from build123d import *

# Parameters (mm, degrees)
SKETCH1_R                 = 2.1
BOSS_EXTRUDE1_DEPTH       = 400
M5X0_8_TAPPED_HOLE1_D     = 4.2
M5X0_8_TAPPED_HOLE1_DEPTH = 14
M5X0_8_TAPPED_HOLE1_TIP   = 1.2618073
M5X0_8_TAPPED_HOLE2_D     = 4.2
M5X0_8_TAPPED_HOLE2_DEPTH = 14
M5X0_8_TAPPED_HOLE2_TIP   = 1.2618073


with BuildPart() as part:
    # Sketch1 → Boss-Extrude1 (new body)
    with BuildSketch(Plane(origin=(0, 0, -400), x_dir=(-1, 0, 0), z_dir=(0, 0, -1))):
        with BuildLine():
            Line((10, -17), (10, -3))
            Line((10, -3), (8, -3))
            Line((8, -3), (8, -6))
            Line((8, -6), (7.060660172, -6))
            Line((7.060660172, -6), (4, -2.939339828))
            Line((4, -2.939339828), (4, -0.519615242))
            Line((4, -0.519615242), (3.7, 0))
            Line((3.7, 0), (4, 0.519615242))
            Line((4, 0.519615242), (4, 2.939339828))
            Line((4, 2.939339828), (7.060660172, 6))
            Line((7.060660172, 6), (8, 6))
            Line((8, 6), (8, 3))
            Line((8, 3), (10, 3))
            Line((10, 3), (10, 17))
            Line((10, 17), (8, 17))
            Line((8, 17), (8, 14))
            Line((8, 14), (7.060660172, 14))
            Line((7.060660172, 14), (4, 17.060660172))
            Line((4, 17.060660172), (4, 19.480384758))
            Line((4, 19.480384758), (3.7, 20))
            Line((3.7, 20), (4, 20.519615242))
            Line((4, 20.519615242), (4, 22.939339828))
            Line((4, 22.939339828), (7.060660172, 26))
            Line((7.060660172, 26), (8, 26))
            Line((8, 26), (8, 23))
            Line((8, 23), (10, 23))
            Line((10, 23), (10, 29))
            ThreePointArc((10, 29), (9.707106781, 29.707106781), (9, 30))
            Line((9, 30), (3, 30))
            Line((3, 30), (3, 28))
            Line((3, 28), (6, 28))
            Line((6, 28), (6, 27.060660172))
            Line((6, 27.060660172), (2.939339828, 24))
            Line((2.939339828, 24), (0.519615242, 24))
            Line((0.519615242, 24), (0, 23.7))
            Line((0, 23.7), (-0.519615242, 24))
            Line((-0.519615242, 24), (-2.939339828, 24))
            Line((-2.939339828, 24), (-6, 27.060660172))
            Line((-6, 27.060660172), (-6, 28))
            Line((-6, 28), (-3, 28))
            Line((-3, 28), (-3, 30))
            Line((-3, 30), (-9, 30))
            ThreePointArc((-9, 30), (-9.707106781, 29.707106781), (-10, 29))
            Line((-10, 29), (-10, 23))
            Line((-10, 23), (-8, 23))
            Line((-8, 23), (-8, 26))
            Line((-8, 26), (-7.060660172, 26))
            Line((-7.060660172, 26), (-4, 22.939339828))
            Line((-4, 22.939339828), (-4, 20.519615242))
            Line((-4, 20.519615242), (-3.7, 20))
            Line((-3.7, 20), (-4, 19.480384758))
            Line((-4, 19.480384758), (-4, 17.060660172))
            Line((-4, 17.060660172), (-7.060660172, 14))
            Line((-7.060660172, 14), (-8, 14))
            Line((-8, 14), (-8, 17))
            Line((-8, 17), (-10, 17))
            Line((-10, 17), (-10, 3))
            Line((-10, 3), (-8, 3))
            Line((-8, 3), (-8, 6))
            Line((-8, 6), (-7.060660172, 6))
            Line((-7.060660172, 6), (-4, 2.939339828))
            Line((-4, 2.939339828), (-4, 0.519615242))
            Line((-4, 0.519615242), (-3.7, 0))
            Line((-3.7, 0), (-4, -0.519615242))
            Line((-4, -0.519615242), (-4, -2.939339828))
            Line((-4, -2.939339828), (-7.060660172, -6))
            Line((-7.060660172, -6), (-8, -6))
            Line((-8, -6), (-8, -3))
            Line((-8, -3), (-10, -3))
            Line((-10, -3), (-10, -17))
            Line((-10, -17), (-8, -17))
            Line((-8, -17), (-8, -14))
            Line((-8, -14), (-7.060660172, -14))
            Line((-7.060660172, -14), (-4, -17.060660172))
            Line((-4, -17.060660172), (-4, -19.480384758))
            Line((-4, -19.480384758), (-3.7, -20))
            Line((-3.7, -20), (-4, -20.519615242))
            Line((-4, -20.519615242), (-4, -22.939339828))
            Line((-4, -22.939339828), (-7.060660172, -26))
            Line((-7.060660172, -26), (-8, -26))
            Line((-8, -26), (-8, -23))
            Line((-8, -23), (-10, -23))
            Line((-10, -23), (-10, -29))
            ThreePointArc((-10, -29), (-9.707106781, -29.707106781), (-9, -30))
            Line((-9, -30), (-3, -30))
            Line((-3, -30), (-3, -28))
            Line((-3, -28), (-6, -28))
            Line((-6, -28), (-6, -27.060660172))
            Line((-6, -27.060660172), (-2.939339828, -24))
            Line((-2.939339828, -24), (-0.519615242, -24))
            Line((-0.519615242, -24), (0, -23.7))
            Line((0, -23.7), (0.519615242, -24))
            Line((0.519615242, -24), (2.939339828, -24))
            Line((2.939339828, -24), (6, -27.060660172))
            Line((6, -27.060660172), (6, -28))
            Line((6, -28), (3, -28))
            Line((3, -28), (3, -30))
            Line((3, -30), (9, -30))
            ThreePointArc((9, -30), (9.707106781, -29.707106781), (10, -29))
            Line((10, -29), (10, -23))
            Line((10, -23), (8, -23))
            Line((8, -23), (8, -26))
            Line((8, -26), (7.060660172, -26))
            Line((7.060660172, -26), (4, -22.939339828))
            Line((4, -22.939339828), (4, -20.519615242))
            Line((4, -20.519615242), (3.7, -20))
            Line((3.7, -20), (4, -19.480384758))
            Line((4, -19.480384758), (4, -17.060660172))
            Line((4, -17.060660172), (7.060660172, -14))
            Line((7.060660172, -14), (8, -14))
            Line((8, -14), (8, -17))
            Line((8, -17), (10, -17))
        make_face()
        Circle(SKETCH1_R, mode=Mode.SUBTRACT)
        with Locations((0, -20)):
            Circle(SKETCH1_R, mode=Mode.SUBTRACT)
        with Locations((0, 20)):
            Circle(SKETCH1_R, mode=Mode.SUBTRACT)
        Polygon((6.939339828, -8), (8, -8), (8, -12), (6.939339828, -12), (2.939339828, -16), (-2.939339828, -16), (-6.939339828, -12), (-8, -12), (-8, -8), (-6.939339828, -8), (-2.939339828, -4), (2.939339828, -4), align=None, mode=Mode.SUBTRACT)
        Polygon((8, 12), (8, 8), (6.939339828, 8), (2.939339828, 4), (-2.939339828, 4), (-6.939339828, 8), (-8, 8), (-8, 12), (-6.939339828, 12), (-2.939339828, 16), (2.939339828, 16), (6.939339828, 12), align=None, mode=Mode.SUBTRACT)
    extrude(amount=-BOSS_EXTRUDE1_DEPTH)

    # M5x0.8 Tapped Hole1
    with Locations(Plane.XY):
        with Locations((0, 20), (0, 0), (0, -20)):
            Hole(M5X0_8_TAPPED_HOLE1_D / 2, depth=M5X0_8_TAPPED_HOLE1_DEPTH)
            with Locations((0, 0, -(M5X0_8_TAPPED_HOLE1_DEPTH + M5X0_8_TAPPED_HOLE1_TIP / 2))):  # 118° drill point
                Cone(0, M5X0_8_TAPPED_HOLE1_D / 2, M5X0_8_TAPPED_HOLE1_TIP, mode=Mode.SUBTRACT)

    # M5x0.8 Tapped Hole2
    with Locations(Plane(origin=(0, 0, -400), x_dir=(-1, 0, 0), z_dir=(0, 0, -1))):
        with Locations((0, -20), (0, 0), (0, 20)):
            Hole(M5X0_8_TAPPED_HOLE2_D / 2, depth=M5X0_8_TAPPED_HOLE2_DEPTH)
            with Locations((0, 0, -(M5X0_8_TAPPED_HOLE2_DEPTH + M5X0_8_TAPPED_HOLE2_TIP / 2))):  # 118° drill point
                Cone(0, M5X0_8_TAPPED_HOLE2_D / 2, M5X0_8_TAPPED_HOLE2_TIP, mode=Mode.SUBTRACT)


solid = part.part
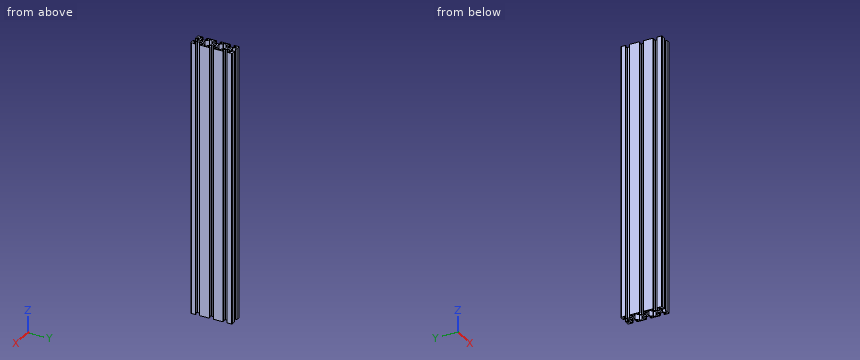
The listing builds one solid part. Answer for the finished solid, in the listing's coordinates (mm). Round coordinates to 2 decimals unless told otherwise and drop trailing zeros. Return JSON: item names as keys, results as strings.
Q1. Find the intervals of material crossed by line 1 along X through (y, z) = (-15, -23); line 2 along Y through (x, z) = (0, -292); line 3 along Y through (x, z) = (-7.5, -56.5), in increasing order. Write a range as from..to.
Results list:
{"line 1": "x = -10..-8, -6.06..-3.94, 3.94..6.06, 8..10", "line 2": "y = -23.7..-22.1, -17.9..-16, -4..-2.1, 2.1..4, 16..17.9, 22.1..23.7", "line 3": "y = -30..-26, -14..-12, -8..-6, 6..8, 12..14, 26..30"}
Q2. Each of these flat-tipped pins is pushed along its axis until it touches: pin 1 Ø2.5 at (y, z) = (18.5, -168) entering from +X; pin 2 Ø3 at (x, z) = (-1, -140) entering from -Y; pin 3 Ø1.8 at (x, z) = (-1.5, -112.5) entering from +Y. Where does it stop, or does it pass through?
Results list:
{"pin 1": "stops at x = 4", "pin 2": "stops at y = -24", "pin 3": "stops at y = 24"}
Q3. Find section A-A, the plane z = -216. State how many separate pieces and enclosed holes the cut face has, plus the area to 3 significant figures.
Results list:
{"separate pieces": "1", "enclosed holes": "5", "area": "465 mm2"}
